```python
from build123d import *

# Parameters (mm, degrees)
BOSS_EXTRUDE3_DEPTH = 3
BOSS_EXTRUDE4_START = 3
BOSS_EXTRUDE4_DEPTH = 10
DRAFT12_ANGLE       = 3
FILLET1_R           = 2
FILLET3_R           = 10
FILLET4_R           = 5
FILLET5_R           = 1


with BuildPart() as part:
    # Sketch2 → Boss-Extrude3 (new body)
    with BuildSketch(Plane(origin=(0, 0, 0), x_dir=(1, 0, 0), z_dir=(0, 1, 0))):
        Polygon((-57.4, 57.4), (-57.4, -57.4), (57.4, -57.4), (57.4, 57.4), (13.13705704, 57.4), (13.13705704, 86.662771881), (-13.13705704, 86.662771881), (-13.13705704, 57.4), align=None)
    extrude(amount=BOSS_EXTRUDE3_DEPTH)

    # Sketch2<5> → Boss-Extrude4 (add)
    with BuildSketch(Plane(origin=(0, 0, 0), x_dir=(1, 0, 0), z_dir=(0, 1, 0)).offset(BOSS_EXTRUDE4_START)):
        Polygon((-57.4, 44.4), (-57.4, -44.4), (-57.4, -57.4), (-44.4, -57.4), (44.4, -57.4), (57.4, -57.4), (57.4, -44.4), (57.4, 44.4), (57.4, 57.4), (44.4, 57.4), (13.13705704, 57.4), (13.13705704, 86.662771881), (-13.13705704, 86.662771881), (-13.13705704, 57.4), (-44.4, 57.4), (-57.4, 57.4), align=None)
        Polygon((54.4, -44.4), (54.4, 44.4), (54.4, 54.4), (44.4, 54.4), (13.13705704, 54.4), (10.13705704, 54.4), (10.13705704, 57.4), (10.13705704, 83.662771881), (-10.13705704, 83.662771881), (-10.13705704, 57.4), (-10.13705704, 54.4), (-13.13705704, 54.4), (-44.4, 54.4), (-54.4, 54.4), (-54.4, 44.4), (-54.4, -44.4), (-54.4, -54.4), (-44.4, -54.4), (44.4, -54.4), (54.4, -54.4), align=None, mode=Mode.SUBTRACT)
    extrude(amount=BOSS_EXTRUDE4_DEPTH)

    # Draft12
    draft12_faces = [part.faces().sort_by_distance(p)[0] for p in [
        (-10.13705704, 8, -69.03138594),
        (-32.26852852, 8, -54.4),
        (-54.4, 8, 0),
        (0, 8, 54.4),
        (54.4, 8, 0),
        (0, 8, -83.662771881),
        (32.26852852, 8, -54.4),
        (10.13705704, 8, -69.03138594),
    ]]
    draft(draft12_faces, Plane.ZX.offset(3), DRAFT12_ANGLE)

    # Fillet1
    fillet1_edges = [part.edges().sort_by_distance(p)[0] for p in [
        (-57.4, 6.5, -57.4),
        (-13.13705704, 6.5, -57.4),
        (-13.13705704, 6.5, -86.662771881),
        (13.13705704, 6.5, -86.662771881),
        (13.13705704, 6.5, -57.4),
        (57.4, 6.5, -57.4),
        (57.4, 6.5, 57.4),
        (-57.4, 6.5, 57.4),
    ]]
    fillet(fillet1_edges, radius=FILLET1_R)

    # Fillet3
    fillet3_edges = [part.edges().sort_by_distance(p)[0] for p in [
        (-54.662038896, 8, -54.662038896),
        (-54.662038896, 8, 54.662038896),
        (54.662038896, 8, 54.662038896),
        (54.662038896, 8, -54.662038896),
    ]]
    fillet(fillet3_edges, radius=FILLET3_R)

    # Fillet4
    fillet4_edges = [part.edges().sort_by_distance(p)[0] for p in [
        (10.399095937, 8, -54.662038896),
        (-10.399095937, 8, -54.662038896),
    ]]
    fillet(fillet4_edges, radius=FILLET4_R)

    # Fillet5
    fillet5_edges = [part.edges().sort_by_distance(p)[0] for p in [
        (10.399095937, 8, -83.924810777),
        (-10.399095937, 8, -83.924810777),
    ]]
    fillet(fillet5_edges, radius=FILLET5_R)


solid = part.part
```
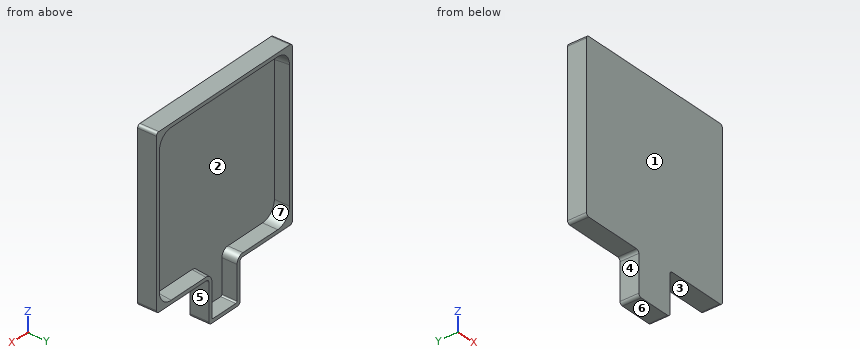
Source: CAD feature listing. Evaluate the final solid. Frame: model axes, mm. Face numbers are marked on the shaded views. A direction names the side the tool comes from. Round coordinates to 2 decimals unless told otherwise and drop trailing zeros. Loops run counter-clockwise (first coordinate to the right, second up) from the corner with the lowest first, then second, coordinate; pieces in that order, holes last. Notation, with made-up numbers: M 21,89.25 L 79,89.25 A14 cw 79,111.25 Z; hole C 48,69.25 d1. An arc over 180 degrees is marked long. Use a Markdown table: item, result. Add a question column.
1. Reachability of the marked faces 1, 2, 3 and 4 from +Z, -Z, +X, -X, +Y, -Y: full face, straight path, thin tool, end or side. Return the list, or none.
2. Section query A-A on x = 36. Return the cut outline in (y, z), then the cut area to 3 significant figures.
3. Mould query, pull axis Z, two halves, no side actions, for the marked faces 5, 6 and 7. Classes: pulls with the +Z half, pulls with the -Z half, needs draft (parallel to the pull), parting line crosses it, or undercut.
4. Line query: line 1 (Z direction, x = 34, y = 12.75); line 2 (Y direction, x = 38, z = -47.5); line 3 (X direction, y = 6.25, z = -3). Output: solid intervals per line, ascending.
5. Contact query for flat-ended pins moving along their axis: P1, Ø2, axis at x = 12, z = -46.5, coming from the +Y side; P2, Ø1.5, axis at x = 2.5, z = 35, coming from the -Y side; P3, Ø6.5, axis at x = 44.5, y = 3.5, coming from the -Z side; P4, Ø6.5, axis at y = 8.5, z = -70, coming from the +X side. Output: stop coordinate, or through.
6. Section query B-B on z = 22. Return the cut outline in (x, y).
Reported:
| question | item | result |
|---|---|---|
| 1 | face 1 | +Z, -Z, +X, -X, -Y |
| 1 | face 2 | +Y |
| 1 | face 3 | -Z, +X, +Y, -Y |
| 1 | face 4 | -Z, -X, +Y, -Y |
| 2 | outline | M 0,-57.4 L 13,-57.4 L 13,-54.92 L 3,-54.4 L 3,54.4 L 13,54.92 L 13,57.4 L 0,57.4 Z |
| 2 | area | 399 mm² |
| 3 | face 5 | needs draft |
| 3 | face 6 | pulls with the -Z half |
| 3 | face 7 | undercut |
| 4 | line 1 | z = -57.4 to -54.91, 54.91 to 57.4 |
| 4 | line 2 | y = 0 to 3 |
| 4 | line 3 | x = -57.4 to -54.57, 54.57 to 57.4 |
| 5 | P1 | stops at y = 3 |
| 5 | P2 | stops at y = 0 |
| 5 | P3 | stops at z = -57.4 |
| 5 | P4 | stops at x = 13.14 |
| 6 | outline | M -57.4,0 L 57.4,0 L 57.4,13 L 54.92,13 L 54.4,3 L -54.4,3 L -54.92,13 L -57.4,13 Z |
